Check sheet for the modelled part. Datum: model origin and axes. Units: mm. A direction names the side the tool comes from. Round coordinates to 2 decimals unless told otherwise and drop trailing zeros. Order: outer loops, then holes, each group sorted by start corner. A loop starts at its lowest first (then second) coordinate and runs counter-clockwise, first axis right, second up. Notation, with made-up numbers: (37.5, 3) -> (50.5, 3) arc R27 ccw to (50.5, 30) -> close; hole circle Ø10 at (2.5, 47). An arc over 180 degrees is marked (long way). Answer in a Markdown table with one row per item.
Autodesk Inventor part; units mm, degrees
ref_plane "YZ Plane" through (0, 0, 0) normal (1, 0, 0) x (0, 1, 0)
ref_plane "XZ Plane" through (0, 0, 0) normal (0, 1, 0) x (-1, 0, 0)
ref_plane "XY Plane" through (0, 0, 0) normal (0, 0, 1) x (1, 0, 0)
sketch "Sketch3" plane through (0, 0, 0) normal (0, 0, 1) x (1, 0, 0)
  line L0 (52.5001, -67.5) -> (-52.5001, -67.5)
  line L1 (-52.5001, -67.5) -> (-52.5001, 67.5)
  line L2 (-52.5001, 67.5) -> (52.5001, 67.5)
  line L3 (52.5001, 67.5) -> (52.5001, -67.5)
  circle A0 centre (32, 32) radius 1.5
  circle A1 centre (-32, 32) radius 1.5
  circle A2 centre (-32, -32) radius 1.5
  circle A3 centre (32, -32) radius 1.5
  line L4 (30.5, 0) -> (-30.5, 0)
  line L5 (30.5, 45) -> (-30.5, 45)
  line L6 (30.5, 45) -> (43.4898, 67.5)
  line L7 (-30.5, 45) -> (-43.4888, 67.5)
  line L8 (30.5, -45) -> (-30.5, -45)
  line L9 (30.5, -45) -> (43.4898, -67.5)
  line L10 (-30.5, -45) -> (-43.4888, -67.5)
  line L11 (0, 42.0002) -> (0, -42)
  line L12 (45, 42.0002) -> (45, -42)
  line L13 (45, 42.0002) -> (52.5001, 54.9914)
  line L14 (45, -42) -> (52.5001, -54.9922)
  line L15 (-45, 42.0002) -> (-45, -42)
  line L16 (-45, 42.0002) -> (-52.5001, 54.9914)
  line L17 (-45, -42) -> (-52.5001, -54.9922)
  circle A4 centre (48, 60.0001) radius 1.428
  circle A5 centre (-48, 60.0001) radius 1.428
  circle A6 centre (48, -59.9999) radius 1.428
  circle A7 centre (-48, -59.9999) radius 1.428
extrude "Extrusion2" add sketch "Sketch3" along normal blind 3 contours L0 L9 L8 L10 L1 L17 L15 L16 L2 L7 L5 L6 L3 L13 L12 L14 | L0 L10 L8 L9 | L14 L12 L13 L3 | L1 L16 L15 L17 | L6 L5 L7 L2 | A4 | A5 | A6 | A7
fillet "Fillet2" radius 4 4 edges at (-52.5001, 67.5, 1.5) (52.5001, 67.5, 1.5) (52.5001, -67.5, 1.5) (-52.5001, -67.5, 1.5)
extrude "Extrusion3" cut sketch "Sketch3" along normal blind 10 contours L0 L10 L8 L9 | L14 L12 L13 L3 | L1 L16 L15 L17 | L6 L5 L7 L2
fillet "Fillet3" radius 10 8 edges at (30.5, 45, 1.5) (-30.5, 45, 1.5) (30.5, -45, 1.5) (-30.5, -45, 1.5) (-52.5001, 54.9914, 1.5) (52.5001, -54.9922, 1.5) (-52.5001, -54.9922, 1.5) (52.5001, 54.9914, 1.5)
fillet "Fillet4" radius 10 4 edges at (45, 42.0002, 1.5) (45, -42, 1.5) (-45, -42, 1.5) (-45, 42.0002, 1.5)
fillet "Fillet5" radius 4 4 edges at (43.4898, 67.5, 1.5) (-43.4888, 67.5, 1.5) (43.4898, -67.5, 1.5) (-43.4888, -67.5, 1.5)
extrude "Extrusion4" cut sketch "Sketch3" along normal blind 10 contours A4 | A5 | A6 | A7
properties part number "GPS - mount v2"
(1) Section check B-B on x = 32. Record the boundary of the cut face in (y, z), plus the area to 3 significant figures.
Solutions:
| item | result |
|---|---|
| outline | (-48.14, 0) -> (-33.5, 0) -> (-33.5, 3) -> (-48.14, 3) -> close; (-30.5, 0) -> (30.5, 0) -> (30.5, 3) -> (-30.5, 3) -> close; (33.5, 0) -> (48.14, 0) -> (48.14, 3) -> (33.5, 3) -> close |
| area | 271 mm^2 |
(2) Scan lines: probe 1 along Y at (x, z) = (32, 1.4); probe 2 along Y at (x, z) = (48, 1.8); probe 3 along X at (y, z) = (-9.5, 0.6). Record each from-to range of solid material in increasing order. Write a range as from..to.
Solutions:
| item | result |
|---|---|
| probe 1 | -48.14..-33.5, -30.5..30.5, 33.5..48.14 |
| probe 2 | -67.5..-61.43, -58.57..-47.2, 47.2..58.57, 61.43..67.5 |
| probe 3 | -45..45 |
(3) Tool access check on faces 4 (the cylindrical face through (-52.17, 55.12, 1.52)), 5 (the cylindrical face through (43.774, -66.949, 1.521)), 6 (the cylindrical face through (43.825, 66.979, 1.521)), 7 (the cylindrical face through (52.15, 55.05, 1.52)), 8 (the cylindrical face through (-51.359, -66.297, 1.521)). Record the directions out of +Z, -Z, +X, -X, +Y, -Y that give a thin tool (end or side, any length) a straight path to the whole face; none if there is none.
Solutions:
| item | result |
|---|---|
| face 4 | +Z, -Z, -X |
| face 5 | +Z, -Z, -Y |
| face 6 | +Z, -Z, +Y |
| face 7 | +Z, -Z, +X |
| face 8 | +Z, -Z, -X, -Y |
(4) Depth check by flat-ended pin: pin 1 Ø1.7 at (x, y) = (48, -60) entering from +Z; pin 2 Ø1.5 at (x, z) = (6.5, 1.5) entering from -Y; pin 3 Ø1.5 at (x, y) = (-26, -27.5) entering from -Z; pin 4 Ø1 at (x, z) = (37, 2.5) entering from +Y. Enter the tip coordinate at first touch or a pass-through.
Solutions:
| item | result |
|---|---|
| pin 1 | through |
| pin 2 | y = -45 |
| pin 3 | z = 0 |
| pin 4 | y = 57.12 |
(5) Section check A-A on y = 32. Record the boundary of the cut face in (x, z), plus the area to 3 significant figures.
Solutions:
| item | result |
|---|---|
| outline | (-45, 0) -> (-33.5, 0) -> (-33.5, 3) -> (-45, 3) -> close; (-30.5, 0) -> (30.5, 0) -> (30.5, 3) -> (-30.5, 3) -> close; (33.5, 0) -> (45, 0) -> (45, 3) -> (33.5, 3) -> close |
| area | 252 mm^2 |
(6) Draft check along Y on faces 1 (the flat face through (-37.798, 57.642, 1.479)), 2 (the flat face through (-52.5, -61, 1)), 3 (the cylindrical face through (-33.2, 32.9, 1.5)). Enter one of: pulls with the +Y half, pulls with the -Y half, needs draft (parallel to the pull), parting line crosses it, or undercut.
Solutions:
| item | result |
|---|---|
| face 1 | pulls with the +Y half |
| face 2 | needs draft |
| face 3 | undercut |
(7) Section check D-D on x = -36.5. Record the boundary of the cut face in (y, z).
Solutions:
| item | result |
|---|---|
| outline | (-55.39, 0) -> (55.39, 0) -> (55.39, 3) -> (-55.39, 3) -> close |
(8) Section check C-C on y = 10.5. Record the boundary of the cut face in (x, z).
Solutions:
| item | result |
|---|---|
| outline | (-45, 0) -> (45, 0) -> (45, 3) -> (-45, 3) -> close |
